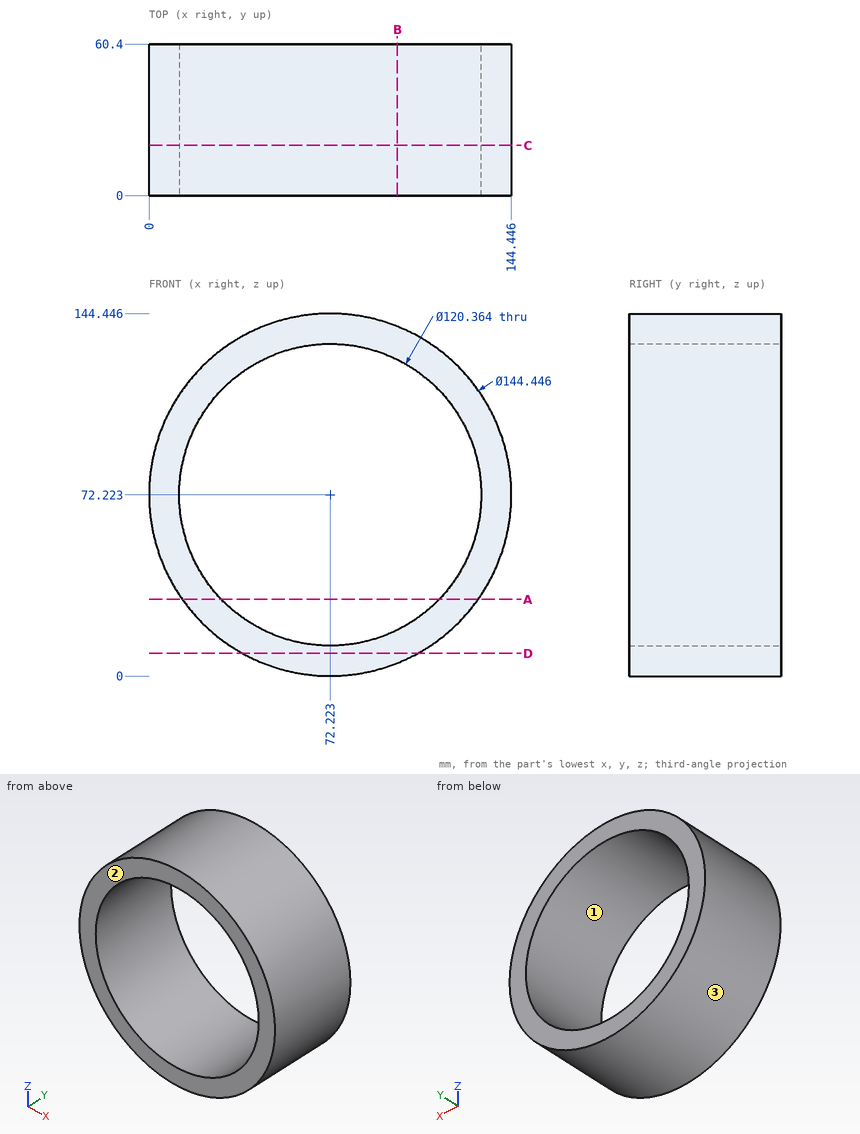
Can you work these out from the drawing? Everything is in mm from the part's minimum corner. Coordinates: 2 decimals unless noted, no trailing zeros. Loops run counter-clockwise (first coordinate to the right, second up) from the corner with the lowest first, then second, coordinate; pieces in that order, holes last.
1) Imagine slicing it at B-B on x = 99. List the corners of the cut face in (y, z) for me.
2) Imagine slicing it at A-A on z = 30.5. List the corners of the cut face in (x, y) for me (1 decimal), plus the area to 3 significant figures.
3) For pin 1 (2 mm diameter, centred on y = 17, z = 73, fed in from +X); pin 2 (1 mm diameter, centred on y = 37, z = 44, fed in from +X); pin 3 (10 mm diameter, centred on x = 77.5, y = 24, fed in from +Z) (1 decimal); pin 4 (2 mm diameter, centred on x = 102, y = 12.5, fed in from -Z), each with a flat end and sliding along its axis, tell me the tip position at first contact or that it passes through.
4) I need wall thicknesses on probe 1 along Z at (x, y) = (104.5, 25) (1 decimal); probe 2 along X at (y, z) = (17.5, 19) (1 decimal); probe 3 along X at (y, z) = (52, 94) (1 decimal). Which ranges of each line are inside material? Lowest first, please.
5) Imagine slicing it at D-D on z = 9. List the corners of the cut face in (x, y) for me, plus the area to 3 significant figures.
6) Thinking about a two-plate mould opening in X: for the marked faces 1, 2 and 3, which applies, pulls with the +X half, pulls with the -X half, needs draft (parallel to the pull), parting line crosses it, or undercut?
7) Imagine slicing it at C-C on y = 20. List the corners of the cut face in (x, z) for me (1 decimal).
Completed:
1. outline: (0, 5.15) - (60.4, 5.15) - (60.4, 18.33) - (0, 18.33) - close; (0, 126.12) - (60.4, 126.12) - (60.4, 139.3) - (0, 139.3) - close
2. outline: (13.3, 0) - (28.9, 0) - (28.9, 60.4) - (13.3, 60.4) - close; (115.6, 0) - (131.2, 0) - (131.2, 60.4) - (115.6, 60.4) - close
2. area: 1,880 mm2
3. pin 1: stops at x = 144.45
3. pin 2: stops at x = 138.91
3. pin 3: stops at z = 144.4
3. pin 4: stops at z = 5.98
4. probe 1: z = 7.6 to 21.4, 123 to 136.8
4. probe 2: x = 23.4 to 44.1, 100.3 to 121
4. probe 3: x = 3.4 to 16.1, 128.3 to 141.1
5. outline: (37.31, 0) - (107.14, 0) - (107.14, 60.4) - (37.31, 60.4) - close
5. area: 4,220 mm2
6. face 1: undercut
6. face 2: needs draft
6. face 3: parting line crosses it
7. outline: circle Ø144.4 at (72.2, 72.2); hole circle Ø120.4 at (72.2, 72.2)
